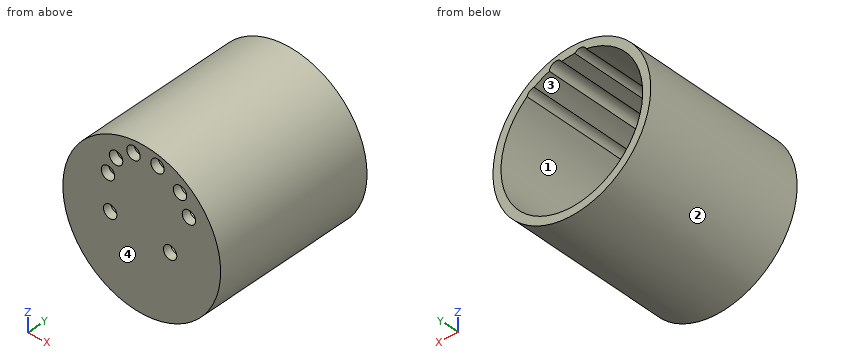
```python
from build123d import *

# Parameters (mm, degrees)
F0_R     = 24.7867182939
F1_DEPTH = 50.8
F2_T     = -2.54
F7_D     = 4.2


# Not quite as in the source:
# - a feature of the source that left no trace in its solid (it failed there, or was rolled back) is left out


with BuildPart() as f1:
    # F0 (on Front) → F1 (new body)
    with BuildSketch(Plane.XZ):
        Circle(F0_R)
    extrude(amount=F1_DEPTH)

    # F2
    f2_openings = [f1.faces().sort_by_distance(p)[0] for p in [
        (0, 0, 0),
    ]]
    offset(amount=F2_T, openings=f2_openings)

    # F7 (through all)
    with Locations(Plane(origin=(0, 0, 0), x_dir=(1, 0, 0), z_dir=(0, 1, 0))):
        with Locations((8.9164366946, 2.3716597352), (14.8237738758, -10.9670488164), (12.0239807293, -16.7495105416), (4.9703707919, -20.9065452218), (-2.5862243492, -20.9065452218), (-8.0531220883, -16.6528206319), (-10.6035573408, -10.9806992114), (-9.9196853116, 0)):
            Hole(F7_D / 2)


solid = f1.part
```
Part model, mm, in its own coordinate system. Face numbers are marked on the shaded views. Round coordinates to 2 decimals unless told otherwise and drop trailing zeros. Loops run counter-clockwise (first coordinate to the right, second up) from the corner with the lowest first, then second, coordinate; pieces in that order, holes last. Notation, with made-up numbers: (-34.5, 53.25) -> (17.5, 53.25) arc R20 ccw to (17.5, 91.25) -> close; hole circle Ø6 at (-18, 43). An arc over 180 degrees is marked (long way). Use one line per item in the form item = value. Start each with the question number.
Item 1: Band-saw the part on B-B (z = -8.5). List the corners of the cut face in (x, y).
Item 2: Band-saw the part on A-A (x = 15.5). List the corners of the cut face in (y, z).
Item 3: Band-saw the part on C-C (y = -10.5). List the corners of the cut face in (x, z).
Item 4: Two-plate mould, pull along X, no slides. Class the marked faces 1, 2, 3 and 4: released by +X, released by -X, zero draft, split by the parting line, or undercut.
Item 5: Band-saw the part on D-D (x = 5). List the corners of the cut face in (y, z), plus the area to 3 significant figures.
Item 6: Drop flat-ended pins along their axis: pin 1 Ø5 at (x, z) = (8.92, -2.37) entering from +Y; pin 2 Ø12 at (y, z) = (-22.5, 16.5) entering from +X; pin 3 Ø5 at (x, y) = (-3.5, -19.5) entering from +Z. Give the stop position or say it passes through.
Item 7: Drill centre lines: line 1 along Z through (x, y) = (0, -5); line 2 along X through (y, z) = (-15, 17); line 3 along Y through (x, z) = (1, 11). Where is each one in solid material? Low to high.
Data:
q1.outline = (-23.28, -50.8) -> (23.28, -50.8) -> (23.28, 0) -> (20.56, 0) -> (20.56, -48.26) -> (-20.56, -48.26) -> (-20.56, 0) -> (-23.28, 0) -> close
q2.outline = (-50.8, -19.34) -> (0, -19.34) -> (0, -15.96) -> (-48.26, -15.96) -> (-48.26, 8.98) -> (-50.8, 8.98) -> close; (-50.8, 12.96) -> (-48.26, 12.96) -> (-48.26, 15.96) -> (0, 15.96) -> (0, 19.34) -> (-50.8, 19.34) -> close
q3.outline = circle Ø49.57 at (0, 0); hole (-4.49, 21.79) arc R22.25 ccw (long way) to (14.07, 17.23) arc R2.1 ccw to (11.83, 18.84) arc R22.25 ccw to (7.06, 21.1) arc R2.1 ccw to (3.19, 22.02) arc R22.25 ccw to (-0.95, 22.23) arc R2.1 ccw to start
q4.face_1 = undercut
q4.face_2 = split by the parting line
q4.face_3 = undercut
q4.face_4 = zero draft
q5.outline = (-50.8, -24.28) -> (0, -24.28) -> (0, -21.68) -> (-48.26, -21.68) -> (-48.26, 18.81) -> (-50.8, 18.81) -> close; (-50.8, 23.01) -> (0, 23.01) -> (0, 24.28) -> (-50.8, 24.28) -> close
q5.area = 299 mm^2
q6.pin_1 = -48.26
q6.pin_2 = 22.45
q6.pin_3 = 24.77
q7.line_1 = -24.79 to -22.25, 22.25 to 24.79
q7.line_2 = -18.04 to -14.35, 14.35 to 18.04
q7.line_3 = -50.8 to -48.26
